```python
from build123d import *

# Parameters (mm, degrees)
F1_DEPTH       = 3
F2_D           = 3.4
F2_CSINK_D     = 6.72
F2_CSINK_ANGLE = 90
F3_SIZE        = 4


with BuildPart() as f1:
    # F0 (on Top) → F1 (new body)
    with BuildSketch(Plane.XY):
        Polygon((31, 21), (-31, 21), (-31, -9), (-21, -9), (-21, -21), (21.0163556039, -21), (21.0163556039, -9), (31, -9), align=None)
        with BuildLine():
            ThreePointArc((17.4355957742, -1.5), (0, -17.5), (-17.4355957742, -1.5))
            Line((-17.4355957742, -1.5), (17.4355957742, -1.5))
        make_face(mode=Mode.SUBTRACT)
        with BuildLine():
            ThreePointArc((-24.4, -4), (-26, -5.6), (-27.6, -4))
            Line((-27.6, -4), (-27.6, 6))
            ThreePointArc((-27.6, 6), (-26, 7.6), (-24.4, 6))
            Line((-24.4, 6), (-24.4, -4))
        make_face(mode=Mode.SUBTRACT)
        with BuildLine():
            Line((17.4355957742, 1.5), (-17.4355957742, 1.5))
            ThreePointArc((-17.4355957742, 1.5), (0, 17.5), (17.4355957742, 1.5))
        make_face(mode=Mode.SUBTRACT)
        with BuildLine():
            ThreePointArc((27.6, -4), (26, -5.6), (24.4, -4))
            Line((24.4, -4), (24.4, 6))
            ThreePointArc((24.4, 6), (26, 7.6), (27.6, 6))
            Line((27.6, 6), (27.6, -4))
        make_face(mode=Mode.SUBTRACT)
    extrude(amount=-F1_DEPTH)

    # F2 (through all)
    with Locations(Plane.XY):
        with Locations((-16.5, 17), (16.5, 17)):
            CounterSinkHole(F2_D / 2, F2_CSINK_D / 2, counter_sink_angle=F2_CSINK_ANGLE)

    # F3
    f3_edges = [f1.edges().sort_by_distance(p)[0] for p in [
        (31, 21, -1.5),
        (-31, 21, -1.5),
    ]]
    chamfer(f3_edges, length=F3_SIZE)

    # F6 (on offset) → F7 section 0
    with BuildSketch(Plane.XY.offset(25)):
        Polygon((-17.9355957742, 1), (-17.9355957742, 8), (-20, 8), (-20, -1), (-17.4355957742, -1), (17.4355957742, -1), (20, -1), (20, 8), (17.9355957742, 8), (17.9355957742, 1), align=None)
    # F4 (on face) → F7 section 1
    with BuildSketch(Plane.XY):
        Polygon((17.4355957742, 1.5), (-17.4355957742, 1.5), (-17.4355957742, 8.5), (-20.5, 8.5), (-20.5, -1.5), (-17.4355957742, -1.5), (17.4355957742, -1.5), (20.5, -1.5), (20.5, 8.5), (17.4355957742, 8.5), align=None)
    loft()


solid = f1.part
```
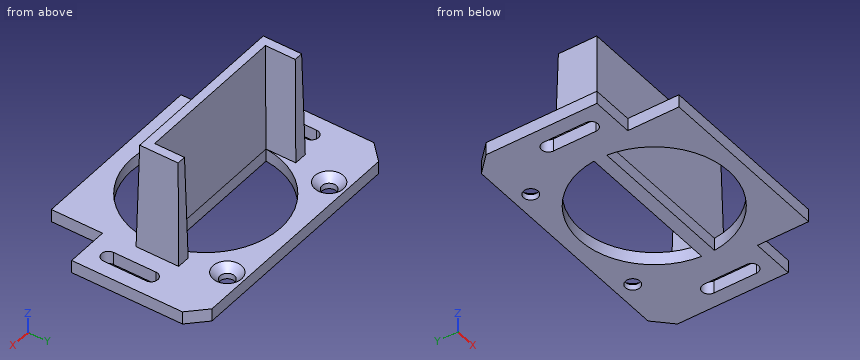
The model under review builds one solid part; all positions refer to its coordinate system, in mm. Round coordinates to 2 decimals unless told otherwise and drop trailing zeros. Loops run counter-clockwise (first coordinate to the right, second up) from the corner with the lowest first, then second, coordinate; pieces in that order, holes last. Notation, with made-up numbers: (57, -26) - (109, -26) arc R29 ccw to (109, -4) - close; hole circle Ø8 at (51, 66). An arc over 180 degrees is marked (long way). Write each question's results on one line, items separated by ' | '. Start each with the question number.
Q1. Take a section at A-A on x = -26. Give the boundary of the cut face in (y, z), plus the area to 3 significant figures.
Q2. Insertion check: P1, Ø3, axis at x = 16.5, y = 17, coming from the +Z side; P2, Ø0.9, axis at x = 23.5, z = -1.5, coming from the -Y side; P3, Ø1.5, axis at y = -12, z = -1, coming from the -X side; P4, Ø2.5, axis at y = -13.5, z = -1, coming from the +X side. Each pin has a flat end and moves straight along its axis. Give the tip position at first contact, or say it passes through.
Q3. Wall thickness on line 1 along X through (y, z) = (7, -1.5); line 2 along Z through (x, y) = (-14.5, 10.5); line 3 along Y through (x, z) = (-2.5, 0.5): over which ranges is each line inside the solid? List them lowest first. Write a range as [from, to].
Q4. Take a section at B-B on z = -1. Give the boundary of the cut face in (x, y).
Q5. Take a section at C-C on x = -1.5. Give the number of separate pieces and of enclosed holes in the cut face, plus the area to 3 significant figures.
Data:
1) outline: (-9, -3) - (-5.6, -3) - (-5.6, 0) - (-9, 0) - close; (7.6, -3) - (21, -3) - (21, 0) - (7.6, 0) - close | area: 50.4 mm²
2) P1: passes through | P2: stops at y = -9 | P3: stops at x = -21 | P4: stops at x = 21.02
3) line 1: x = [-31, -27.25], [-24.75, -16.04], [16.04, 24.75], [27.25, 31] | line 2: z = [-3, 0] | line 3: y = [-1.49, 1.49]
4) outline: (-31, -9) - (-21, -9) - (-21, -21) - (21.02, -21) - (21.02, -9) - (31, -9) - (31, 17) - (27, 21) - (-27, 21) - (-31, 17) - close; hole (-27.6, -4) arc R1.6 ccw to (-24.4, -4) - (-24.4, 6) arc R1.6 ccw to (-27.6, 6) - close; hole circle Ø4.72 at (-16.5, 17); hole (-17.44, -1.5) arc R17.5 ccw to (17.44, -1.5) - close; hole (-17.44, 1.5) - (17.44, 1.5) arc R17.5 ccw to start; hole circle Ø4.72 at (16.5, 17); hole (24.4, -4) arc R1.6 ccw to (27.6, -4) - (27.6, 6) arc R1.6 ccw to (24.4, 6) - close
5) separate pieces: 3 | enclosed holes: 0 | area: 92.9 mm²
